Geometry: final body of the model. Coordinates: model frame, mm. Face numbers are marked on the shaded views. A direction names the side the tool comes from. Give positions to 0.01 mm unless a question says otherwise; leave off trailing zeros. Write each loop counter-clockwise with the first axis right and the second up, starting at its lowest first coordinate (ties: lowest second). Pieces come first, ordered by that corner, then holes. Notation, with made-up numbers: M 1,40 L 50,40 A21 ccw 50,62 Z; hole C 47.5,-38.5 d1. An arc over 180 degrees is marked long. Use a Markdown table: item, result. Add a question column.
1) Line query: line 1 (X direction, y = 8, z = 40); line 2 (Z direction, x = 129, y = 0.5); line 3 (Z direction, x = 105, y = -2.75). Output: solid intervals per line, ascending.
2) Section D-D on z = 27. Return the cut outline in (x, y).
3) Pin query (flat end, axial travel): pin 1 (6 mm diameter, centred on y = 6.5, z = 13.5, fed in from -X); pin 2 (8 mm diameter, centred on x = 154.5, y = -4.5, fed in from -Z); pin 3 (8 mm diameter, centred on x = 40, z = 15.5, fed in from +Y); pin 4 (2 mm diameter, centred on y = 7, z = 3, fed in from -X). Return the tip coordinate at first contact, or that it passes through.
4) Set-up query: the marked faces 1 and 2. Return all of +Z, -Z, +X, -X, +Y, -Y with unobstructed straight access to the full face (end or side cutting, diameter ignored); none if empty.
5) Section C-C on x = 46. Return the cut outline in (y, z), then the cut area to 3 significant figures.
6) Section B-B on y = 0. Return the cut outline in (x, z).
7) Section A-A on z = 8. Return the cut outline in (x, y).
```python
from build123d import *

# Parameters (mm, degrees)
SKETCH_1_R      = 10
EXTRUDE_1_DEPTH = 200
SKETCH_4_W      = 8.886532998
SKETCH_4_H      = 20
EXTRUDE_2_DEPTH = 67


with BuildPart() as part:
    # 草图1 → 凸台-拉伸1 (new body)
    with BuildSketch(Plane(origin=(0, 0, 0), x_dir=(0, 0, -1), z_dir=(1, 0, 0))):
        Circle(SKETCH_1_R)
    extrude(amount=EXTRUDE_1_DEPTH)

    # 草图4 → 凸台-拉伸2 (add)
    with BuildSketch(Plane.XY):
        with Locations((100.138852078, 0)):
            Rectangle(SKETCH_4_W, SKETCH_4_H)
    extrude(amount=EXTRUDE_2_DEPTH)


solid = part.part
```
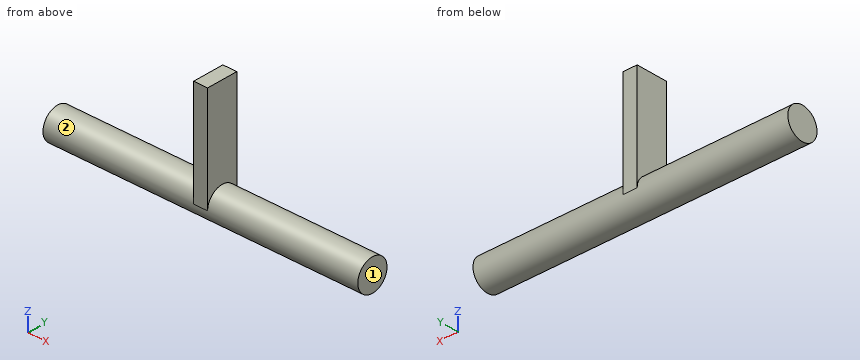
Found:
| question | item | result |
|---|---|---|
| 1 | line 1 | 95.7 to 104.58 |
| 1 | line 2 | -9.99 to 9.99 |
| 1 | line 3 | -9.61 to 9.61 |
| 2 | outline | M 95.7,-10 L 104.58,-10 L 104.58,10 L 95.7,10 Z |
| 3 | pin 1 | x = 95.7 |
| 3 | pin 2 | z = -9.99 |
| 3 | pin 3 | through |
| 3 | pin 4 | x = 0 |
| 4 | face 1 | +Z, -Z, +X, +Y, -Y |
| 4 | face 2 | none |
| 5 | outline | C 0,0 d20 |
| 5 | area | 314 mm² |
| 6 | outline | M 0,-10 L 200,-10 L 200,10 L 104.58,10 L 104.58,67 L 95.7,67 L 95.7,10 L 0,10 Z |
| 7 | outline | M 0,-6 L 95.7,-6 L 95.7,-10 L 104.58,-10 L 104.58,-6 L 200,-6 L 200,6 L 104.58,6 L 104.58,10 L 95.7,10 L 95.7,6 L 0,6 Z |
